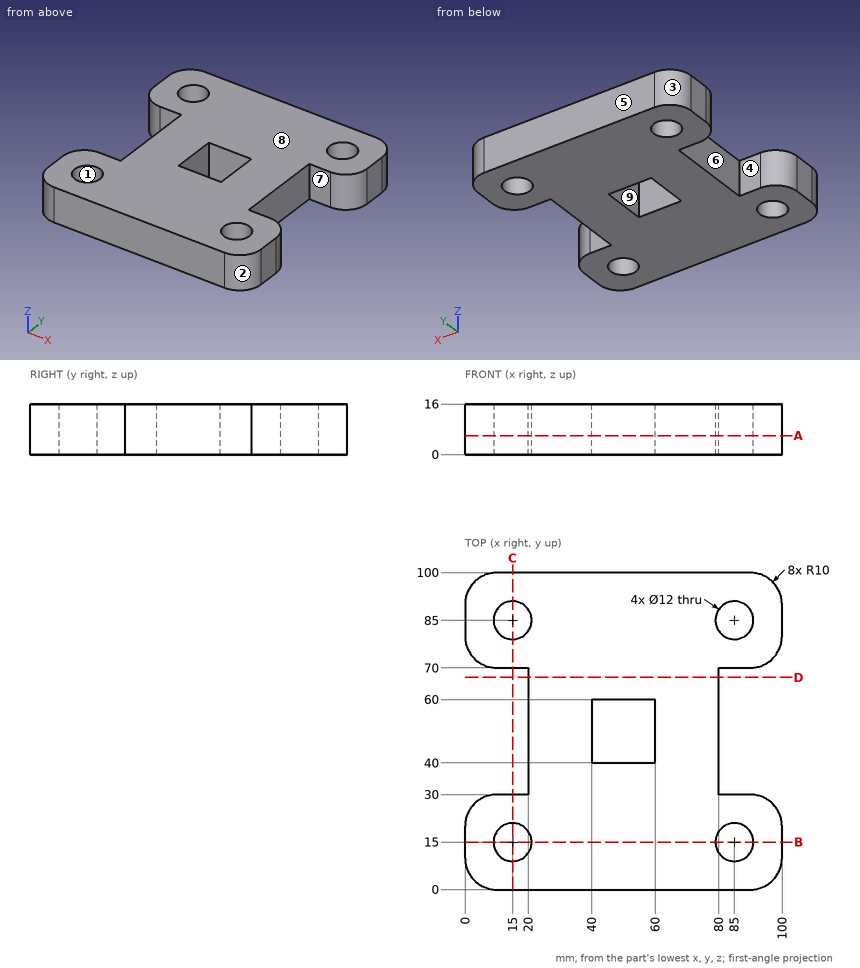
Design review of the part shown in the three views and the two pictorial views. Dimensions are in mm from the part's minimum x, y and z. A direction names the side the tool comes from. Give positions to 0.01 mm unless a question says otherwise; leave off trailing zeros. Write each loop counter-clockwise with the first axis right and the second up, starting at its lowest first coordinate (ties: lowest second). Pieces come first, ordered by that corner, then holes. Notation, with made-up numbers: M 53,71.5 L 112,71.5 A31 ccw 112,99.5 Z; hole C 0.5,71.25 d9. An arc over 180 degrees is marked long. Answer in a Markdown table with one row per item.
Item 1: Tool access review of the marked faces 5, 6, 7, 8 and 9: name each direction out of +Z, -Z, +X, -X, +Y, -Y from which nothing blocks a thin tool from reaching the whole face with its end or side.
Check sheet entries:
| item | result |
|---|---|
| face 5 | +Z, -Z, +X, -X, +Y |
| face 6 | +Z, -Z, -X |
| face 7 | +Z, -Z, +X |
| face 8 | +Z, +X, -X, +Y, -Y |
| face 9 | +Z, -Z |
Item 2: Add section C-C on x = 15. Give the boundary of the cut face in (y, z).
Check sheet entries:
| item | result |
|---|---|
| outline | M 0,0 L 9,0 L 9,16 L 0,16 Z; M 21,0 L 30,0 L 30,16 L 21,16 Z; M 70,0 L 79,0 L 79,16 L 70,16 Z; M 91,0 L 100,0 L 100,16 L 91,16 Z |
Item 3: Add section B-B on y = 15. Give the boundary of the cut face in (x, z), plus the area to 3 significant figures.
Check sheet entries:
| item | result |
|---|---|
| outline | M 0,0 L 9,0 L 9,16 L 0,16 Z; M 21,0 L 79,0 L 79,16 L 21,16 Z; M 91,0 L 100,0 L 100,16 L 91,16 Z |
| area | 1,220 mm2 |
Item 4: For P1, Ø8, axis at y = 51, z = 4.5, coming from the +X side; P2, Ø8, axis at y = 50.5, z = 11.5, coming from the -X side, all flat-tipped, find the tip position at first contact; note any pin that passes through.
Check sheet entries:
| item | result |
|---|---|
| P1 | x = 80 |
| P2 | x = 20 |
Item 5: For line 1 along Y through (x, z) = (15, 9); line 2 along X through (y, z) = (85.5, 12.75); line 3 along Y through (x, z) = (57, 12.75), list the stretches that pass through material, from the lowest coordinate up.
Check sheet entries:
| item | result |
|---|---|
| line 1 | 0 to 9, 21 to 30, 70 to 79, 91 to 100 |
| line 2 | 0 to 9.02, 20.98 to 79.02, 90.98 to 100 |
| line 3 | 0 to 40, 60 to 100 |
Item 6: Add section A-A on z = 6. Give the boundary of the cut face in (x, y), plus the area to 3 significant figures.
Check sheet entries:
| item | result |
|---|---|
| outline | M 0,10 A10 ccw 10,0 L 90,0 A10 ccw 100,10 L 100,20 A10 ccw 90,30 L 80,30 L 80,70 L 90,70 A10 ccw 100,80 L 100,90 A10 ccw 90,100 L 10,100 A10 ccw 0,90 L 0,80 A10 ccw 10,70 L 20,70 L 20,30 L 10,30 A10 ccw 0,20 Z; hole C 15,15 d12; hole C 15,85 d12; hole M 40,40 L 60,40 L 60,60 L 40,60 Z; hole C 85,15 d12; hole C 85,85 d12 |
| area | 7,380 mm2 |
Item 7: Add section D-D on y = 67. Give the boundary of the cut face in (x, z), plus the area to 3 significant figures.
Check sheet entries:
| item | result |
|---|---|
| outline | M 20,0 L 80,0 L 80,16 L 20,16 Z |
| area | 960 mm2 |
Item 8: Draft analysis for pull direction Y (two halves, no side actions). For the marked faces 1, 2, 3 and 4, state which applies: +Y half, -Y half, draft (parallel to the pull), parting line (faces both ways), or undercut.
Check sheet entries:
| item | result |
|---|---|
| face 1 | undercut |
| face 2 | -Y half |
| face 3 | +Y half |
| face 4 | undercut |
